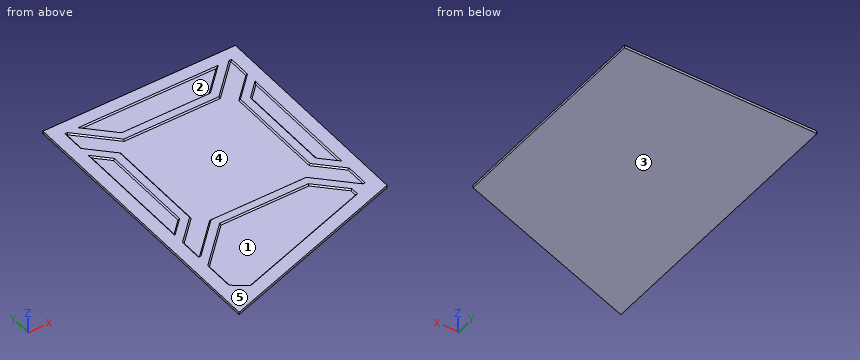
```python
from build123d import *

# Parameters (mm, degrees)
BOSS_EXTRU_1_DEPTH      = 10
ENL_V_MAT_EXTRU_1_DEPTH = 5
CHANFREIN1_SIZE         = 5


with BuildPart() as part:
    # Esquisse1 → Boss.-Extru.1 (new body)
    with BuildSketch(Plane.XY):
        Polygon((750, 0), (0, -250), (0, 0), (0, 850), (750, 850), align=None)
    extrude(amount=BOSS_EXTRU_1_DEPTH)

    # Esquisse2 → Enlèv. mat.-Extru.1 (cut)
    with BuildSketch(Plane.XY.offset(10)):
        Polygon((110, 241.923881554), (110, 608.076118446), (50, 668.076118446), (50, 181.923881554), align=None)
        Polygon((201.923881554, 700), (548.076118446, 700), (648.076118446, 800), (101.923881554, 800), align=None)
        Polygon((50, 800), (50, 710.502525317), (140, 620.502525317), (140, 229.497474683), (50, 139.497474683), (50, 50), (59.497474683, 50), (189.497474683, 180), (560.502525317, 180), (690.502525317, 50), (700, 50), (700, 139.497474683), (610, 229.497474683), (610, 620.502525317), (700, 710.502525317), (700, 800), (690.502525317, 800), (560.502525317, 670), (189.497474683, 670), (59.497474683, 800), align=None)
        Polygon((700, 668.076118446), (700, 181.923881554), (640, 241.923881554), (640, 608.076118446), align=None)
        Polygon((648.076118446, 50), (548.076118446, 150), (201.923881554, 150), (101.923881554, 50), (50, -1.923881554), (50, -120.628705664), (106.920997883, -161.655039703), (648.076118446, 18.730000485), align=None)
    extrude(amount=-ENL_V_MAT_EXTRU_1_DEPTH, mode=Mode.SUBTRACT)

    # Chanfrein1
    chanfrein1_edges = [part.edges().sort_by_distance(p)[0] for p in [
        (50, 425, 5),
        (80, 638.076118446, 5),
        (124.497474683, 735, 5),
        (375, 670, 5),
        (140, 425, 5),
        (95, 665.502525317, 5),
        (50, 755.251262658, 5),
        (54.748737342, 800, 5),
        (375, 800, 5),
        (375, 700, 5),
        (151.923881554, 750, 5),
        (110, 425, 5),
        (80, 211.923881554, 5),
        (625.502525317, 735, 5),
        (695.251262658, 800, 5),
        (700, 755.251262658, 5),
        (655, 665.502525317, 5),
        (610, 425, 5),
        (655, 184.497474683, 5),
        (700, 94.748737342, 5),
        (695.251262658, 50, 5),
        (625.502525317, 115, 5),
        (375, 180, 5),
        (124.497474683, 115, 5),
        (54.748737342, 50, 5),
        (50, 94.748737342, 5),
        (95, 184.497474683, 5),
        (598.076118446, 750, 5),
        (700, 425, 5),
        (670, 211.923881554, 5),
        (640, 425, 5),
        (670, 638.076118446, 5),
        (375, 150, 5),
        (598.076118446, 100, 5),
        (648.076118446, 34.365000242, 5),
        (377.498558164, -71.462519609, 5),
        (78.460498942, -141.141872683, 5),
        (50, -61.276293609, 5),
        (125.961940777, 74.038059223, 5),
    ]]
    chamfer(chanfrein1_edges, length=CHANFREIN1_SIZE - 0.0001)  # a hair under: the kernel refuses the full size


solid = part.part
```
Work out the finished part from the listing and answer in its coordinate system (mm). Face numbers are marked on the shaded views. A direction names the side the tool comes from. Give positions to 0.01 mm unless a question says otherwise; leave off trailing zeros. Return JSON: item names as keys, results as strings.
1) Straight lines are drawn through the part: line 1 along Y through (x, z) = (423, 9.25); line 2 along Y through (x, z) = (210, 8); line 3 along X through (y, z) = (482, 9.5). For each, find the intervals that lie inside material, in ascending order. Write a range as [from, to].
Resolved:
{"line 1": "[-109, -55.5], [149.25, 180.75], [669.25, 700.75], [799.25, 850]", "line 2": "[-180, -125.19], [148, 182], [668, 702], [798, 850]", "line 3": "[0, 50.5], [109.5, 140.5], [609.5, 640.5], [699.5, 750]"}
2) This flat-tipped pin is pushed along its axis until it touches: pin 1 (12 mm diameter, centred on x = 622.5, y = -53.5, fed in from +Z). Where does it stop, or does it pass through?
Resolved:
{"pin 1": "through"}
3) A tool of negligible diameter and unlimited length cuts with its end or side. For the marked faces 4 and 5, from which of +Z, -Z, +X, -X, +Y, -Y can it reach the whole face along a straight path? Write none if from no direction.
Resolved:
{"face 4": "+Z", "face 5": "+Z, +X, -X, +Y, -Y"}
4) For a pull along X with two mould halves and no side action, classify the marked faces 1, 2 and 3 as +X half, -X half, draft (parallel to the pull), parting line (faces both ways), or undercut.
Resolved:
{"face 1": "undercut", "face 2": "undercut", "face 3": "draft"}
5) Section C-C, the plane z = 8 is taken. Give the number of separate pieces and of enclosed holes in the cut face, plus the area to 3 significant figures.
Resolved:
{"separate pieces": "1", "enclosed holes": "5", "area": "261,000 mm^2"}
